Could you check a few things on this drawing? It's one solid part, dimensions in mm from its lowest x, y, z. A direction names the side the tool comes from. Round coordinates to 2 decimals unless told otherwise and drop trailing zeros. Write each loop counter-clockwise with the first axis right and the second up, starting at its lowest first coordinate (ties: lowest second). Pieces come first, ordered by that corner, then holes. Notation, with made-up numbers: (1, 56.25) - (52, 56.25) arc R19 cw to (52, 77.25) - close; hole circle Ø11 at (82.5, 17). An arc over 180 degrees is marked (long way). One line per question, with ' | ' between items. Start each with the question number.
(1) Thinking about a two-plate mould opening in Y: for the marked faces 1, 2 and 3, which applies, pulls with the +Y half, pulls with the -Y half, needs draft (parallel to the pull), parting line crosses it, or undercut?
(2) If I drill on L1, parallel to X at y = 21, z = 2.25; L2, parallel to Y at x = 21, z = 1.55, over which ranges is the centre line in solid material (lowest first)?
(3) For the marked faces 4 and 5, which set-ups out of +Z, -Z, +X, -X, +Y, -Y let a thin tool reach every point of the face, with its end or its side?
(4) Will these pins go through, and if not, where does the flat tip stop? pin 1 (3 mm diameter, centred on x = 28.5, z = 2.5, fed in from +Y); pin 2 (6 mm diameter, centred on x = 21, y = 21, fed in from +Z); pin 3 (1.5 mm diameter, centred on y = 36, z = 6.5, fed in from +X).
(5) Imagine slicing it at A-A (y = 21). Write out the boundary of the cut face in (x, z), plus the area to 3 significant figures.
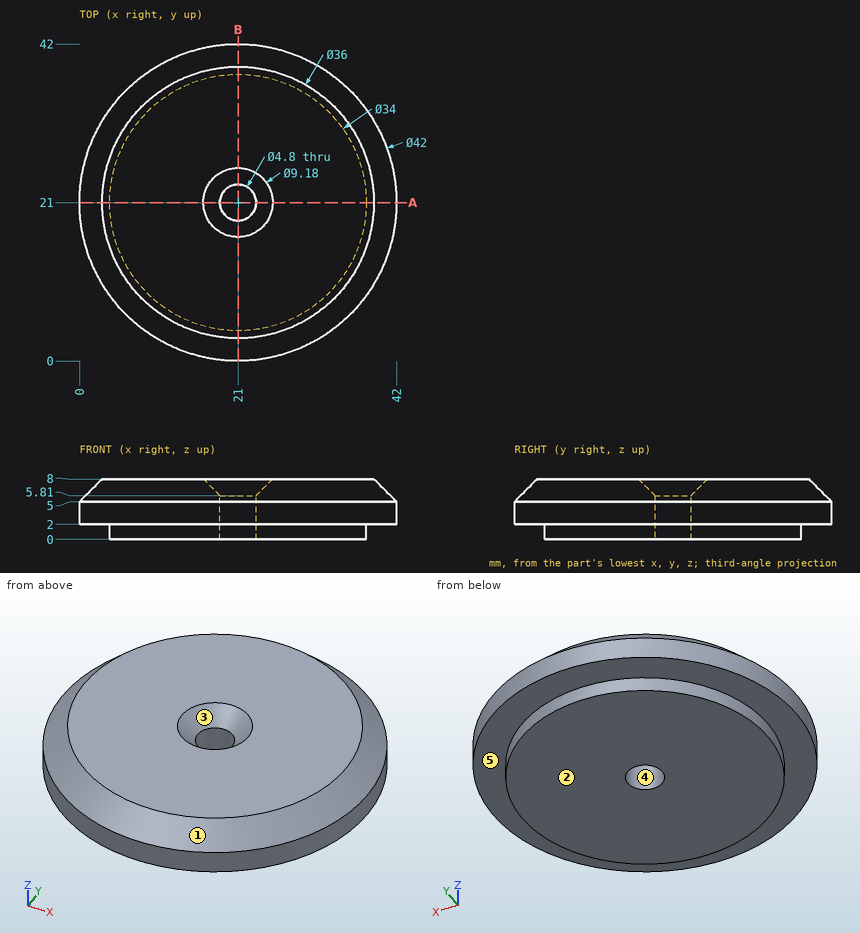
Check sheet entries:
1) face 1: parting line crosses it | face 2: needs draft | face 3: undercut
2) L1: 0 to 18.6, 23.4 to 42 | L2: 4 to 18.6, 23.4 to 38
3) face 4: +Z, -Z | face 5: -Z
4) pin 1: y = 41.12 | pin 2: z = 6.41 | pin 3: x = 34.87
5) outline: (0, 2) - (4, 2) - (4, 0) - (18.6, 0) - (18.6, 5.81) - (16.41, 8) - (3, 8) - (0, 5) - close; (23.4, 0) - (38, 0) - (38, 2) - (42, 2) - (42, 5) - (39, 8) - (25.59, 8) - (23.4, 5.81) - close | area: 268 mm^2
